For this review, use the dimensioned drawing (mm, ordinates from the lowest corner) and the shaded views. A direction names the side the tool comes from. Coordinates: 2 decimals unless noted, no trailing zeros. Loops run counter-clockwise (first coordinate to the right, second up) from the corner with the lowest first, then second, coordinate; pieces in that order, holes last.
1. Take a section at A-A, the plane y = 13.95. State the section outline as (x, z) points.
2. Take a section at C-C, the plane z = 24.5. State the section outline as (x, y) points.
3. To check wall thickness, follow probe 1 along Z at (x, y) = (18, 2.5); probe 2 along Z at (x, y) = (23.25, 9.75); probe 3 along X at (y, z) = (14, 18.5). State the ranges of each line that lie inside material, in increasing order.
4. Take a section at B-B, the plane z = 6. State the section outline as (x, y) points, then the cut area to 3 significant figures.
5. Machinability: for the marked faces 1 and 2, which of the approach directions +Z, -Z, +X, -X, +Y, -Y give a long, thin tool a straight path to every point of the face, cutting with its end or side? Answer none if there is none.
6. Clearance check with flat-ended pins moving along their axes: P1, Ø1.5, axis at x = 22.5, y = 19.5, coming from the +Z side; P2, Ø1.8, axis at x = 16.54, y = 21.52, coming from the -Z side; P3, Ø5, axis at y = 12, z = 16.5, coming from the +X side. State where each tip first meets the part, or that it passes through.
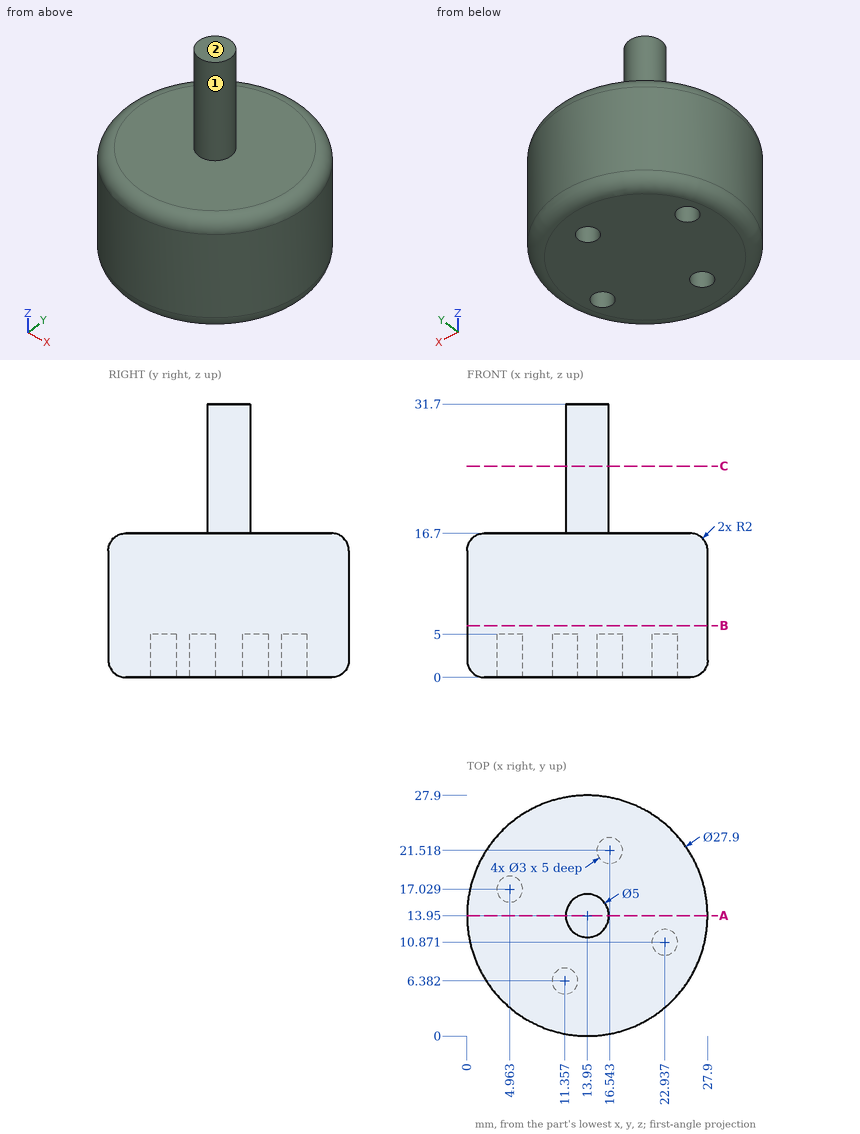
Results list:
1. outline: (0, 2) arc R2 ccw to (2, 0) - (25.9, 0) arc R2 ccw to (27.9, 2) - (27.9, 14.7) arc R2 ccw to (25.9, 16.7) - (16.45, 16.7) - (16.45, 31.7) - (11.45, 31.7) - (11.45, 16.7) - (2, 16.7) arc R2 ccw to (0, 14.7) - close
2. outline: circle Ø5 at (13.95, 13.95)
3. probe 1: z = 0.01 to 16.69
3. probe 2: z = 5 to 16.7
3. probe 3: x = 11.45 to 16.45
4. outline: circle Ø27.9 at (13.95, 13.95)
4. area: 611 mm2
5. face 1: +Z
5. face 2: +Z, +X, -X, +Y, -Y
6. P1: stops at z = 16.7
6. P2: stops at z = 5
6. P3: stops at x = 27.9
